Model file for the job. Use its own axes, mm. A direction names the side the tool comes from. Coordinates: 2 decimals unless noted, no trailing zeros. Order: outer loops, then holes, each group sorted by start corner. A loop starts at its lowest first (then second) coordinate and runs counter-clockwise, first axis right, second up. Notation, with made-up numbers: M -20,-16 L -6,-16 A15 ccw -6,-1 Z; hole C 89.5,10.5 d5. An arc over 180 degrees is marked long. Return JSON: item names as keys, results as strings.
```python
from build123d import *

# Parameters (mm, degrees)
SKETCH1_W               = 25.4
SKETCH1_H               = 25.4
BOSS_EXTRUDE1_DEPTH     = 38.1
SHELL1_T                = -1.5875
CUT_EXTRUDE1_DEPTH      = 43.121134838
CUT_EXTRUDE1_DEPTH_BACK = 43.121134838
SKETCH2_R               = 2.4892
SKETCH3_R               = 2.4892
CUT_EXTRUDE2_DEPTH      = 48.519048812


with BuildPart() as part:
    # Sketch1 → Boss-Extrude1 (new, symmetric)
    with BuildSketch(Plane.XY):
        Rectangle(SKETCH1_W, SKETCH1_H)
    extrude(amount=BOSS_EXTRUDE1_DEPTH, both=True)

    # Shell1
    shell1_openings = [part.faces().sort_by_distance(p)[0] for p in [
        (0, 0, 38.1),
        (0, 0, -38.1),
    ]]
    offset(amount=SHELL1_T, openings=shell1_openings, kind=Kind.INTERSECTION)

    # Sketch2 → Cut-Extrude1 (cut, two sides: drawn at the far end of the back side and taken through both)
    with BuildSketch(Plane(origin=(0, 0, 0), x_dir=(1, 0, 0), z_dir=(0, 1, 0)).offset(-CUT_EXTRUDE1_DEPTH_BACK)):
        with Locations(Location((0, -25.4, 0), (0, 0, 270))):
            Circle(SKETCH2_R)
        with Locations(Location((0, -12.7, 0), (0, 0, 270))):
            Circle(SKETCH2_R)
        with Locations(Location((0, 0, 0), (0, 0, 270))):
            Circle(SKETCH2_R)
        with Locations(Location((0, 12.7, 0), (0, 0, 270))):
            Circle(SKETCH2_R)
        with Locations(Location((0, 25.4, 0), (0, 0, 270))):
            Circle(SKETCH2_R)
    extrude(amount=CUT_EXTRUDE1_DEPTH + CUT_EXTRUDE1_DEPTH_BACK, mode=Mode.SUBTRACT)

    # Sketch3 → Cut-Extrude2 (cut, through all)
    with BuildSketch(Plane.ZY.offset(12.7)):
        with Locations((-25.4, 0)):
            Circle(SKETCH3_R)
        with Locations((-12.7, 0)):
            Circle(SKETCH3_R)
        Circle(SKETCH3_R)
        with Locations((12.7, 0)):
            Circle(SKETCH3_R)
        with Locations((25.4, 0)):
            Circle(SKETCH3_R)
    extrude(amount=-CUT_EXTRUDE2_DEPTH, mode=Mode.SUBTRACT)


solid = part.part
```
Item 1: 3-axis set-ups, long thin cutter, end or side, ignore diameter. For faces 1 (the flat face through (-12.7, 3, 1)), 2 (the flat face through (11.112, -3, 1)): which of +Z, -Z, +X, -X, +Y, -Y reach the whole face in a straight line?
Check result:
{"face 1": "+Z, -Z, -X, +Y, -Y", "face 2": "+Z, -Z"}
Item 2: Wall check: line 1 (Z direction, x = 0, y = 12.35); line 2 (Y direction, x = 6.75, z = 15.5); line 3 (X direction, y = -11.9, z = -12.7). Give the ranges that are in metal, low to high.
Check result:
{"line 1": "z = -38.1 to -27.89, -22.91 to -15.19, -10.21 to -2.49, 2.49 to 10.21, 15.19 to 22.91, 27.89 to 38.1", "line 2": "y = -12.7 to -11.11, 11.11 to 12.7", "line 3": "x = -12.7 to -2.49, 2.49 to 12.7"}
Item 3: Saw through at B-B (z = 25.4). Write the cut outline in (x, y).
Check result:
{"outline": "M -12.7,-12.7 L -2.49,-12.7 L -2.49,-11.11 L -11.11,-11.11 L -11.11,-2.49 L -12.7,-2.49 Z; M -12.7,2.49 L -11.11,2.49 L -11.11,11.11 L -2.49,11.11 L -2.49,12.7 L -12.7,12.7 Z; M 2.49,-12.7 L 12.7,-12.7 L 12.7,-2.49 L 11.11,-2.49 L 11.11,-11.11 L 2.49,-11.11 Z; M 2.49,11.11 L 11.11,11.11 L 11.11,2.49 L 12.7,2.49 L 12.7,12.7 L 2.49,12.7 Z"}
Item 4: Pull direction Z, two halves, no side cores. Call faces 3 (the cylindrical face through (-11.917, 0.748, -10.326)), 4 (the flat face through (-11.3, 0.1, -38.1)), 5 (the cylindrical face through (-11.917, 0.748, 2.374)), 6 (the flat face through (-3, -11.112, 1)): +Z half, -Z half, draft (parallel to the pull), parting line (faces both ways), or undercut.
Check result:
{"face 3": "undercut", "face 4": "-Z half", "face 5": "undercut", "face 6": "draft"}
Item 5: Drop a flat-ended pin along its axis: pin 1 Ø3 at (x, z) = (0, -12.7) entering from -Y. Give the stop position or say it passes through.
Check result:
{"pin 1": "passes through"}
Item 6: Saw through at D-D (z = -8). Write the cut outline in (x, y), and give its area (3 significant figures).
Check result:
{"outline": "M -12.7,-12.7 L 12.7,-12.7 L 12.7,12.7 L -12.7,12.7 Z; hole M -11.11,-11.11 L 11.11,-11.11 L 11.11,11.11 L -11.11,11.11 Z", "area": "151 mm2"}
Item 7: Saw through at A-A (y = 6). Write the cut outline in (x, z).
Check result:
{"outline": "M -12.7,-38.1 L -11.11,-38.1 L -11.11,38.1 L -12.7,38.1 Z; M 11.11,-38.1 L 12.7,-38.1 L 12.7,38.1 L 11.11,38.1 Z"}
